```python
from build123d import *

# Parameters (mm, degrees)
SKETCH1_W               = 100
SKETCH1_H               = 100
BASE_FLANGE1_DEPTH      = 1.5875
EDGE_FLANGE1_DEPTH      = 100
EDGE_FLANGE2_DEPTH      = 100
F_1_4_CLEARANCE_HOLE1_D = 6.7564


# Sheet-metal steps are written as plain solids
with BuildPart() as part:
    # Sketch1 → Base-Flange1 (new body)
    with BuildSketch(Plane(origin=(0, 0, 0), x_dir=(1, 0, 0), z_dir=(0, 1, 0))):
        Rectangle(SKETCH1_W, SKETCH1_H)
    extrude(amount=-BASE_FLANGE1_DEPTH)

    # Edge-Flange1 section (across the edge) → Edge-Flange1 (add)
    with BuildSketch(Plane(origin=(-53.2, 0, -50), x_dir=(1, 0, 0), z_dir=(0, 0, 1))):
        with BuildLine():
            Line((-1.5875, 3.2), (-1.5875, 98.4125))
            Line((-1.5875, 98.4125), (0, 98.4125))
            Line((0, 98.4125), (0, 3.2))
            ThreePointArc((0, 3.2), (0.9372583, 0.9372583), (3.2, 0))
            Line((3.2, 0), (3.2, -1.5875))
            ThreePointArc((3.2, -1.5875), (-0.185273715, -0.185273715), (-1.5875, 3.2))
        make_face()
    extrude(amount=EDGE_FLANGE1_DEPTH)

    # Edge-Flange2 section (across the edge) → Edge-Flange2 (add)
    with BuildSketch(Plane(origin=(-50, 0, 53.2), x_dir=(0, 0, -1), z_dir=(1, 0, 0))):
        with BuildLine():
            Line((-1.5875, 3.2), (-1.5875, 98.4125))
            Line((-1.5875, 98.4125), (0, 98.4125))
            Line((0, 98.4125), (0, 3.2))
            ThreePointArc((0, 3.2), (0.9372583, 0.9372583), (3.2, 0))
            Line((3.2, 0), (3.2, -1.5875))
            ThreePointArc((3.2, -1.5875), (-0.185273715, -0.185273715), (-1.5875, 3.2))
        make_face()
    extrude(amount=EDGE_FLANGE2_DEPTH)

    # 1/4 Clearance Hole1 (through all)
    with Locations(Plane(origin=(0, 0, 0), x_dir=(1, 0, 0), z_dir=(0, 1, 0))):
        with Locations((-30, -5), (30, -5)):
            Hole(F_1_4_CLEARANCE_HOLE1_D / 2)


solid = part.part
```
CAD build for the part. Positions are in the model's coordinates, mm. A direction names the side the tool comes from. Give positions to 0.01 mm unless a question says otherwise; leave off trailing zeros. Loops run counter-clockwise (first coordinate to the right, second up) from the corner with the lowest first, then second, coordinate; pieces in that order, holes last. Notation, with made-up numbers: (72.25, -37.75) - (77.25, -37.75) arc R10 ccw to (77.25, -29.75) - close; hole circle Ø3 at (42, 19). An arc over 180 degrees is marked (long way). Put each result on its own line as item: value.
Q1. Probe line 1 along Z through (x, y) = (20, 21); line 2 along Y through (x, z) = (11, -44); line 3 along X through (y, z) = (86, 14.5). List the from-to ranges inside material, lowest first.
Filled in:
line 1: z = 53.2 to 54.79
line 2: y = -1.59 to 0
line 3: x = -54.79 to -53.2
Q2. Flat gauge pins, fed straight in: pin 1 (3 mm diameter, centred on x = -19, y = 29, fed in from -Z); pin 2 (1.5 mm diameter, centred on y = 29, z = 16.5, fed in from +X); pin 3 (5 mm diameter, centred on x = 28, z = -9.5, fed in from +Y); pin 4 (5.5 mm diameter, centred on x = 30, z = 5, fed in from +Y). Where does each tip first touch, or does it go through?
Filled in:
pin 1: stops at z = 53.2
pin 2: stops at x = -53.2
pin 3: stops at y = 0
pin 4: passes through
Q3. Slice it at C-C (x = -30). Give the cut face in (y, z) (1 decimal).
Filled in:
outline: (-1.6, -50) - (0, -50) - (0, 1.6) - (-1.6, 1.6) - close; (-1.6, 8.4) - (0, 8.4) - (0, 50) arc R3.2 cw to (3.2, 53.2) - (98.4, 53.2) - (98.4, 54.8) - (3.2, 54.8) arc R4.8 ccw to (-1.6, 50) - close
Q4. Slice it at D-D (z = 19). Give the cut face in (x, y) (1 decimal).
Filled in:
outline: (-54.8, 3.2) arc R4.8 ccw to (-50, -1.6) - (50, -1.6) - (50, 0) - (-50, 0) arc R3.2 cw to (-53.2, 3.2) - (-53.2, 98.4) - (-54.8, 98.4) - close
Q5. Mould opens along Z. For faces 6 (the face through (26.879, -0.805, 6.294)), 7 (the face through (-1, 50, 54.788)), 8 (the face through (-1, -1.588, -1)), 9 (the face through (-33.222, -0.805, 3.985)) say: pulls with the +Z half, pulls with the -Z half, needs draft (parallel to the pull), parting line crosses it, or undercut.
Filled in:
face 6: undercut
face 7: pulls with the +Z half
face 8: needs draft
face 9: undercut
Q6. Tool access for faces 1 (the face through (-53.2, 51, -1)), 2 (the face through (-1, 51, 53.2)), 3 (the face through (-53.35, -0.22, -0.7)), 4 (the face through (-1, 0, -1)), 5 (the face through (-0.7, -0.22, 53.35)): list every direction of +Z, -Z, +X, -X, +Y, -Y with a clear straight run to the whole face (end or side of a thin tool).
Filled in:
face 1: +Z, -Z, +X, +Y
face 2: -Z, +X, -X, +Y
face 3: +Z, -Z, -X, -Y
face 4: -Z, +X, +Y
face 5: +Z, +X, -X, -Y
Q7. Slice it at B-B (z = 5). Give the cut face in (x, y) (1 decimal), plus the area to 3 significant figures.
Filled in:
outline: (-54.8, 3.2) arc R4.8 ccw to (-50, -1.6) - (-33.4, -1.6) - (-33.4, 0) - (-50, 0) arc R3.2 cw to (-53.2, 3.2) - (-53.2, 98.4) - (-54.8, 98.4) - close; (-26.6, -1.6) - (26.6, -1.6) - (26.6, 0) - (-26.6, 0) - close; (33.4, -1.6) - (50, -1.6) - (50, 0) - (33.4, 0) - close
area: 298 mm²
Q8. Slice it at A-A (y = 89). Give the cut face in (x, z), plus the area to 4 significant figures.
Filled in:
outline: (-54.79, -50) - (-53.2, -50) - (-53.2, 50) - (-54.79, 50) - close; (-50, 53.2) - (50, 53.2) - (50, 54.79) - (-50, 54.79) - close
area: 317.5 mm²
